Read the model definition and answer for the solid it produces. Units are mm, in the model's axes. A direction names the side the tool comes from. Round coordinates to 2 decimals unless told otherwise and drop trailing zeros. Order: outer loops, then holes, each group sorted by start corner. A loop starts at its lowest first (then second) coordinate and runs counter-clockwise, first axis right, second up. Notation, with made-up numbers: (67.5, 0) - (97.5, 0) arc R20 cw to (97.5, 5) - close; hole circle Ø1 at (23, 66.5). An arc over 180 degrees is marked (long way). Put each result on its own line as item: value. Start each with the question number.
Q1. Which of the six approach directions +Z, -Z, +X, -X, +Y, -Y give full straight-line access (tool end or side, diameter ignored) to faces 4 (the face through (8.874, 0.11, 26.248)), 5 (the face through (3, 9.3, -6.2)), 6 (the face through (13.944, -5.362, -12.932))?
Q2. Section A-A on z = 0 is taken. Give the vertices of the cut face in (x, y), then the cut area to 3 significant figures.
Q3. For a pull along Z with two mould halves and no side action, classify faces 1 (the face through (8.874, -10.916, -26.327)), 2 (the face through (0, -6, 13)), 3 (the face through (8.874, -20.458, -9.377)) as pulls with the +Z half, pulls with the -Z half, needs draft (parallel to the pull), parting line crosses it, or undercut.
Q4. Each of these flat-tipped pins is pushed along its axis until it touches: pin 1 Ø1 at (x, z) = (8, 20) entering from -Y; pin 2 Ø8 at (x, z) = (16, -12) entering from +Y; pin 3 Ø25 at (y, z) = (0, 0) entering from -X. Where does it stop, or does it pass through?
Q5. Section C-C on y = 19.5 is taken. Give the vertices of the cut face in (x, z), then the cut area to 4 significant figures.
Q6. Find the intervals of material crossed by line 1 along Y through (x, z) = (5.75, 0); line 2 along Z through (x, y) = (16, 0.5); line 3 along Z through (x, y) = (7, -2), in increasing order. Write a range as from..to.
Q7. Section D-D on x = 12.5 is taken. Give the vertices of the cut face in (y, z) (3 decimals).
Q8. Section B-B on y = 0 is taken. Give the vertices of the cut face in (x, z).
from build123d import *

# Parameters (mm, degrees)
SKETCH1_R           = 28.5
SKETCH1_R_2         = 11
SKETCH1_R_3         = 2.5
BOSS_EXTRUDE1_DEPTH = 18
CUT_EXTRUDE1_START  = -8
SKETCH2_R           = 14
SKETCH2_R_2         = 11
CUT_EXTRUDE1_DEPTH  = 8
SKETCH3_R           = 14
SKETCH3_R_2         = 11
CUT_EXTRUDE2_DEPTH  = 3


with BuildPart() as part:
    # Sketch1 → Boss-Extrude1 (new body)
    with BuildSketch(Plane(origin=(0, 0, 0), x_dir=(0, 0, -1), z_dir=(1, 0, 0))):
        Circle(SKETCH1_R)
        Circle(SKETCH1_R_2, mode=Mode.SUBTRACT)
        with Locations((-23.75, 0)):
            Circle(SKETCH1_R_3, mode=Mode.SUBTRACT)
        with Locations((-11.875, 20.56810334)):
            Circle(SKETCH1_R_3, mode=Mode.SUBTRACT)
        with Locations((11.875, 20.56810334)):
            Circle(SKETCH1_R_3, mode=Mode.SUBTRACT)
        with Locations((23.75, 0)):
            Circle(SKETCH1_R_3, mode=Mode.SUBTRACT)
        with Locations((11.875, -20.56810334)):
            Circle(SKETCH1_R_3, mode=Mode.SUBTRACT)
        with Locations((-11.875, -20.56810334)):
            Circle(SKETCH1_R_3, mode=Mode.SUBTRACT)
    extrude(amount=BOSS_EXTRUDE1_DEPTH)

    # Sketch2 → Cut-Extrude1 (cut)
    with BuildSketch(Plane(origin=(18, 0, 0), x_dir=(0, 0, -1), z_dir=(1, 0, 0)).offset(CUT_EXTRUDE1_START)):
        Circle(SKETCH2_R)
        Circle(SKETCH2_R_2, mode=Mode.SUBTRACT)
    extrude(amount=CUT_EXTRUDE1_DEPTH, mode=Mode.SUBTRACT)

    # Sketch3 → Cut-Extrude2 (cut)
    with BuildSketch(Plane.ZY):
        with Locations(Location((0, 0, 0), (0, 0, 180))):
            Circle(SKETCH3_R)
        Circle(SKETCH3_R_2, mode=Mode.SUBTRACT)
    extrude(amount=-CUT_EXTRUDE2_DEPTH, mode=Mode.SUBTRACT)


solid = part.part
Findings:
1. face 4: +X, -X
1. face 5: -X
1. face 6: +X
2. outline: (0, -28.5) - (18, -28.5) - (18, -14) - (10, -14) - (10, -11) - (3, -11) - (3, -14) - (0, -14) - close; (0, 14) - (3, 14) - (3, 11) - (10, 11) - (10, 14) - (18, 14) - (18, 28.5) - (0, 28.5) - close
2. area: 564 mm2
3. face 1: parting line crosses it
3. face 2: needs draft
3. face 3: undercut
4. pin 1: y = -20.78
4. pin 2: y = 27.35
4. pin 3: x = 3
5. outline: (0, -20.78) - (18, -20.78) - (18, -14.14) - (0, -14.14) - close; (0, -9.61) - (18, -9.61) - (18, 9.61) - (0, 9.61) - close; (0, 14.14) - (18, 14.14) - (18, 20.78) - (0, 20.78) - close
5. area: 585.5 mm2
6. line 1: -28.5..-11, 11..28.5
6. line 2: -28.5..-26.2, -21.3..-13.99, 13.99..21.3, 26.2..28.5
6. line 3: -28.43..-25.25, -22.25..-10.82, 10.82..22.25, 25.25..28.43
7. outline: circle Ø57 at (0, 0); hole circle Ø5 at (-20.568, -11.875); hole circle Ø5 at (-20.568, 11.875); hole circle Ø28 at (0, 0); hole circle Ø5 at (0, -23.75); hole circle Ø5 at (0, 23.75); hole circle Ø5 at (20.568, -11.875); hole circle Ø5 at (20.568, 11.875)
8. outline: (0, -28.5) - (18, -28.5) - (18, -26.25) - (0, -26.25) - close; (0, -21.25) - (18, -21.25) - (18, -14) - (10, -14) - (10, -11) - (3, -11) - (3, -14) - (0, -14) - close; (0, 14) - (3, 14) - (3, 11) - (10, 11) - (10, 14) - (18, 14) - (18, 21.25) - (0, 21.25) - close; (0, 26.25) - (18, 26.25) - (18, 28.5) - (0, 28.5) - close
